Build history of the part. All positions in model axes, mm. Round coordinates to 2 decimals unless told otherwise and drop trailing zeros. Write each loop counter-clockwise with the first axis right and the second up, starting at its lowest first coordinate (ties: lowest second). Pieces come first, ordered by that corner, then holes.
Item 1: Band-saw the part on C-C, the plane z = -60.5. Write the cut outline in (x, y).
Item 2: Band-saw the part on A-A, the plane x = 2.5. Count the separate pieces of the cut face and the enclosed holes in it, then the cut area to 3 significant figures.
Item 3: Wall check: probe 1 along Z at (x, y) = (1.2, -230); probe 2 along Z at (x, y) = (1.8, -44.5); probe 3 along Y at (x, z) = (1.4, -20). Give the ranges that are in metal, low to high.
Item 4: Band-saw the part on D-D, the plane z = 0. Write the cut outline in (x, y).
Item 5: Band-saw the part on B-B, the plane y = 0. Write the cut outline in (x, z).
Item 6: Drop flat-ended pins along their axis: pin 1 Ø1.5 at (x, y) = (2, -89) entering from -Z; pin 2 Ø4 at (y, z) = (-230, -32.5) entering from -X; pin 3 Ø3 at (x, y) = (1, -23) entering from -Z. Give the stop position or say it passes through.
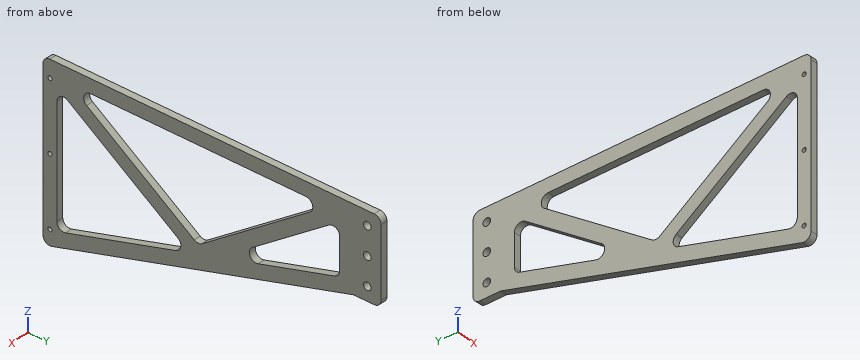
```python
from build123d import *

# Parameters (mm, degrees)
SKETCH1_R            = 1.5
BOSS_EXTRUDE1_DEPTH  = 5
M5_CLEARANCE_HOLE1_D = 5.5
FILLET2_R            = 5


with BuildPart() as part:
    # Sketch1 → Boss-Extrude1 (new body)
    with BuildSketch(Plane(origin=(0, 0, 0), x_dir=(0, 0, -1), z_dir=(1, 0, 0))):
        Polygon((95, -235), (30, -10), (30, 10), (-30, 10), (-30, -235), align=None)
        with Locations((-17.5, -230)):
            Circle(SKETCH1_R, mode=Mode.SUBTRACT)
        with Locations((32.5, -230)):
            Circle(SKETCH1_R, mode=Mode.SUBTRACT)
        with Locations((82.5, -230)):
            Circle(SKETCH1_R, mode=Mode.SUBTRACT)
        Polygon((-13.887165787, -225), (53.870859832, -128.66078689), (81.702188063, -225), align=None, mode=Mode.SUBTRACT)
        Polygon((-20, -216.308695426), (-20, -28.691304574), (45.978242739, -122.5), align=None, mode=Mode.SUBTRACT)
        Polygon((22.479965841, -20), (47.830060977, -107.750329315), (-13.887165787, -20), align=None, mode=Mode.SUBTRACT)
    extrude(amount=BOSS_EXTRUDE1_DEPTH)

    # M5 Clearance Hole1 (through all)
    with Locations(Plane(origin=(5, 0, 0), x_dir=(0, 0, -1), z_dir=(1, 0, 0))):
        with Locations((0, 0), (20, 0), (-20, 0)):
            Hole(M5_CLEARANCE_HOLE1_D / 2)

    # Fillet2
    fillet2_edges = [part.edges().sort_by_distance(p)[0] for p in [
        (2.5, -235, -95),
        (2.5, -235, 30),
        (2.5, 10, 30),
        (2.5, 10, -30),
        (2.5, -10, -30),
        (2.5, -216.308695426, 20),
        (2.5, -122.5, -45.978242739),
        (2.5, -28.691304574, 20),
        (2.5, -20, -22.479965841),
        (2.5, -20, 13.887165787),
        (2.5, -107.750329315, -47.830060977),
        (2.5, -225, 13.887165787),
        (2.5, -225, -81.702188063),
        (2.5, -128.66078689, -53.870859832),
    ]]
    fillet(fillet2_edges, radius=FILLET2_R)


solid = part.part
```
Results:
1. outline: (0, -235) - (5, -235) - (5, -225) - (0, -225) - close; (0, -151.61) - (5, -151.61) - (5, -115.58) - (0, -115.58) - close
2. separate pieces: 1
2. enclosed holes: 9
2. area: 9,790 mm2
3. probe 1: z = -93.35 to -84, -81 to -34, -31 to 16, 19 to 30
3. probe 2: z = -39.97 to -29.56, -3.34 to 8.88, 20 to 30
3. probe 3: y = -235 to -225, -176.82 to -159.44, -85.56 to -68.18, -20.17 to -2.75, 2.75 to 10
4. outline: (0, -235) - (5, -235) - (5, -225) - (0, -225) - close; (0, -205.26) - (5, -205.26) - (5, -187.87) - (0, -187.87) - close; (0, -57.13) - (5, -57.13) - (5, -39.74) - (0, -39.74) - close; (0, -20) - (5, -20) - (5, -2.75) - (0, -2.75) - close; (0, 2.75) - (5, 2.75) - (5, 10) - (0, 10) - close
5. outline: (0, -30) - (5, -30) - (5, -22.75) - (0, -22.75) - close; (0, -17.25) - (5, -17.25) - (5, -2.75) - (0, -2.75) - close; (0, 2.75) - (5, 2.75) - (5, 17.25) - (0, 17.25) - close; (0, 22.75) - (5, 22.75) - (5, 30) - (0, 30) - close
6. pin 1: stops at z = -53.04
6. pin 2: stops at x = 0
6. pin 3: stops at z = -34.19
